```python
from build123d import *

# Parameters (mm, degrees)
SKETCH1_R           = 9.9
BOSS_EXTRUDE1_DEPTH = 1.5
SKETCH2_R           = 5.1
BOSS_EXTRUDE2_DEPTH = 4.5
SKETCH3_R           = 3.5
CUT_EXTRUDE1_DEPTH  = 7


with BuildPart() as part:
    # Sketch1 → Boss-Extrude1 (new body)
    with BuildSketch(Plane.XY.offset(28.963778517)):
        with Locations((13.758033718, 17.384066602)):
            Circle(SKETCH1_R)
    extrude(amount=BOSS_EXTRUDE1_DEPTH)

    # Sketch2 → Boss-Extrude2 (add)
    with BuildSketch(Plane(origin=(0, 0, 28.963778517), x_dir=(-1, 0, 0), z_dir=(0, 0, -1))):
        with Locations((-13.758033718, 17.384066602)):
            Circle(SKETCH2_R)
    extrude(amount=BOSS_EXTRUDE2_DEPTH)

    # Sketch3 → Cut-Extrude1 (cut, through all)
    with BuildSketch(Plane(origin=(0, 0, 24.463778517), x_dir=(-1, 0, 0), z_dir=(0, 0, -1))):
        with Locations((-13.758033718, 17.384066602)):
            Circle(SKETCH3_R)
    extrude(amount=-CUT_EXTRUDE1_DEPTH, mode=Mode.SUBTRACT)


solid = part.part
```
Verification items for the finished model (mm, model axes). A direction names the side the tool comes from. Coordinates: 2 decimals unless noted, no trailing zeros. Loops run counter-clockwise (first coordinate to the right, second up) from the corner with the lowest first, then second, coordinate; pieces in that order, holes last. Notation, with made-up numbers: (19.25, 44) -> (57.25, 44) arc R17 cw to (57.25, 67) -> close; hole circle Ø2 at (-28, 64.25). An arc over 180 degrees is marked (long way). Put each result on its own line as item: value.
1. Section check B-B, the plane x = 14.75. Record the boundary of the cut face in (y, z).
Result set:
outline: (7.53, 28.96) -> (12.38, 28.96) -> (12.38, 24.46) -> (14.03, 24.46) -> (14.03, 30.46) -> (7.53, 30.46) -> close; (20.74, 24.46) -> (22.39, 24.46) -> (22.39, 28.96) -> (27.23, 28.96) -> (27.23, 30.46) -> (20.74, 30.46) -> close
2. Mould release check, pull along Y, two halves, no side actions. Record for faces 1 (the face through (16.338, 19.75, 27.422)), 2 (the face through (17.805, 14.281, 26.745)), 3 (the face through (18, 18, 30.464)): pulls with the +Y half, pulls with the -Y half, needs draft (parallel to the pull), parting line crosses it, or undercut.
Result set:
face 1: undercut
face 2: parting line crosses it
face 3: needs draft
3. Gauge pin test, flat ends, axial feed: P1, Ø1, axis at x = 8, y = 23.5, coming from the -Z side; P2, Ø6, axis at x = 9, y = 15, coming from the -Z side; P3, Ø5.5, axis at x = 13.76, y = 17.38, coming from the +Z side; P4, Ø3, axis at y = 22.5, z = 25.5, coming from the -X side. Record the tip position at first contact, or that the pin passes through.
Result set:
P1: stops at z = 28.96
P2: stops at z = 24.46
P3: passes through
P4: stops at x = 10.16
4. Section check A-A, the plane y = 20.5. Record the boundary of the cut face in (x, z), then the cut area to 3 significant figures.
Result set:
outline: (4.36, 28.96) -> (9.72, 28.96) -> (9.72, 24.46) -> (12.16, 24.46) -> (12.16, 30.46) -> (4.36, 30.46) -> close; (15.35, 24.46) -> (17.8, 24.46) -> (17.8, 28.96) -> (23.15, 28.96) -> (23.15, 30.46) -> (15.35, 30.46) -> close
area: 45.4 mm^2
5. Tool access check on faces 4 (the face through (11, 22, 28.964)), 5 (the face through (6.461, 24.075, 29.703)). Record the directions out of +Z, -Z, +X, -X, +Y, -Y that give a thin tool (end or side, any length) a straight path to the whole face; none if there is none.
Result set:
face 4: -Z
face 5: +Z, -Z
6. Thickness scan on line 1 (X direction, y = 17.25, z = 29.9); line 2 (Z direction, x = 22, y = 14.75); line 3 (Y direction, x = 16, z = 30.1). Record the ranges inside material, lowest first.
Result set:
line 1: x = 3.86 to 10.26, 17.26 to 23.66
line 2: z = 28.96 to 30.46
line 3: y = 7.74 to 14.7, 20.07 to 27.03
7. Section check C-C, the plane x = 17.5. Record the boundary of the cut face in (y, z).
Result set:
outline: (8.22, 28.96) -> (13.92, 28.96) -> (13.92, 24.46) -> (20.85, 24.46) -> (20.85, 28.96) -> (26.55, 28.96) -> (26.55, 30.46) -> (8.22, 30.46) -> close
8. Section check D-D, the plane z = 26.7. Record the boundary of the cut face in (x, y), then the cut area to 3 significant figures.
Result set:
outline: circle Ø10.2 at (13.76, 17.38); hole circle Ø7 at (13.76, 17.38)
area: 43.2 mm^2
